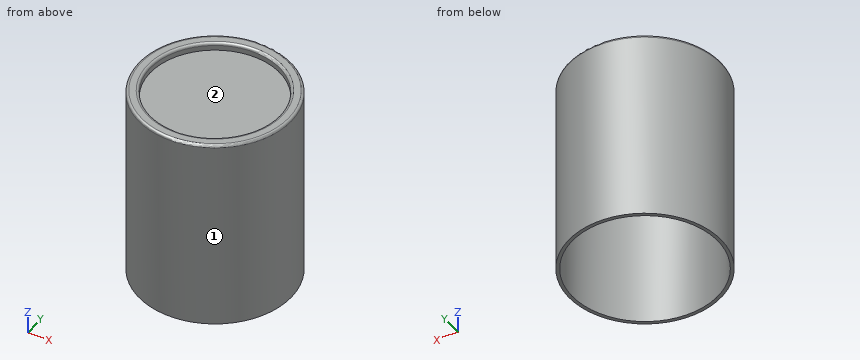
```python
from build123d import *

# Parameters (mm, degrees)
F0_R     = 30
F1_DEPTH = 73
F2_DEPTH = 3.5
F5_D     = 51
F5_DEPTH = 3.5
F5_TIP   = 15.3219457852
F6_R     = 1
F7_T     = -1.3


with BuildPart() as f1:
    # F0 (on Top) → F1 (new body)
    with BuildSketch(Plane.XY):
        Circle(F0_R)
    extrude(amount=F1_DEPTH)

    # F2 (add): a face of the model
    f2_faces = [f1.faces().sort_by_distance(p)[0] for p in [
        (0, 0, 73),
    ]]
    extrude(f2_faces, amount=F2_DEPTH)

    # F5 (one way)
    with BuildSketch(Plane(origin=(0, 0, 73.5), x_dir=(1, 0, 0), z_dir=(0, 0, -1))):
        with Locations((0, 0)):
            Circle(F5_D / 2)
    extrude(amount=-F5_DEPTH, mode=Mode.SUBTRACT)
    with Locations(Plane(origin=(0, 0, 73.5), x_dir=(1, 0, 0), z_dir=(0, 0, -1))):
        with Locations((0, 0)):
            with Locations((0, 0, -(F5_DEPTH + F5_TIP / 2))):  # 118° drill point
                Cone(0, F5_D / 2, F5_TIP, mode=Mode.SUBTRACT)

    # F6
    f6_edges = [f1.edges().sort_by_distance(p)[0] for p in [
        (-30, 0, 76.5),
        (-25.5, 0, 76.5),
    ]]
    fillet(f6_edges, radius=F6_R)

    # F7
    f7_openings = [f1.faces().sort_by_distance(p)[0] for p in [
        (0, 0, 0),
    ]]
    offset(amount=F7_T, openings=f7_openings, kind=Kind.INTERSECTION)


solid = f1.part
```
Here's how the part is built. I have some questions about the finished solid (model axes, mm). Face numbers are marked on the shaded views. Coordinates: 2 decimals unless noted, no trailing zeros. Order: outer loops, then holes, each group sorted by start corner. A loop starts at its lowest first (then second) coordinate and runs counter-clockwise, first axis right, second up. Notation, with made-up numbers: M -32,-25.5 L -5,-25.5 A13 ccw -5,-15.5 Z; hole C -27,24.5 d10. An arc over 180 degrees is marked long. Answer as a JSON object with one key per item and string values. Group by question number.
(1) If we mould it in two halves opening along X, with no side actions, what happens to the marked faces 1 and 2? For each: released by +X, released by -X, zero draft, split by the parting line, or undercut.
(2) Suppose I cut it at C-C, the plane z = 27. Please give me the cut outline in (x, y).
(3) I need wall thicknesses on probe 1 along Y at (x, z) = (0, 73.95); probe 2 along Y at (x, z) = (0, 25); probe 3 along Z at (x, y) = (-18, -20). Which ranges of each line are inside material? Lowest first, please.
(4) For pin 1 (15.5 mm diameter, centred on x = -12.5, y = -10, fed in from +Z); pin 2 (2 mm diameter, centred on x = 10.5, z = 65.5, fed in from -Y); pin 3 (16 mm diameter, centred on x = 5, y = 2.5, fed in from -Z), each with a flat end and sliding along its axis, tell me the tip position at first contact or that it passes through.
(5) Suppose I cut it at A-A, the plane y = 0. Please give me the cut outline in (x, z), then the cut area to 3 significant figures.
Values found:
{
 "1": {"face 1": "split by the parting line", "face 2": "undercut"},
 "2": {"outline": "C 0,0 d60; hole C 0,0 d57.4"},
 "3": {"probe 1": "y = -30 to -28.7, -26.8 to -25.5, 25.5 to 26.8, 28.7 to 30", "probe 2": "y = -30 to -28.7, 28.7 to 30", "probe 3": "z = 75.2 to 76.5"},
 "4": {"pin 1": "stops at z = 73.5", "pin 2": "stops at y = -28.46", "pin 3": "stops at z = 72.2"},
 "5": {"outline": "M -30,0 L -28.7,0 L -28.7,75.2 L -26.8,75.2 L -26.8,72.2 L 26.8,72.2 L 26.8,75.2 L 28.7,75.2 L 28.7,0 L 30,0 L 30,75.5 A1 ccw 29,76.5 L 26.5,76.5 A1 ccw 25.5,75.5 L 25.5,73.5 L -25.5,73.5 L -25.5,75.5 A1 ccw -26.5,76.5 L -29,76.5 A1 ccw -30,75.5 Z", "area": "280 mm^2"}
}
